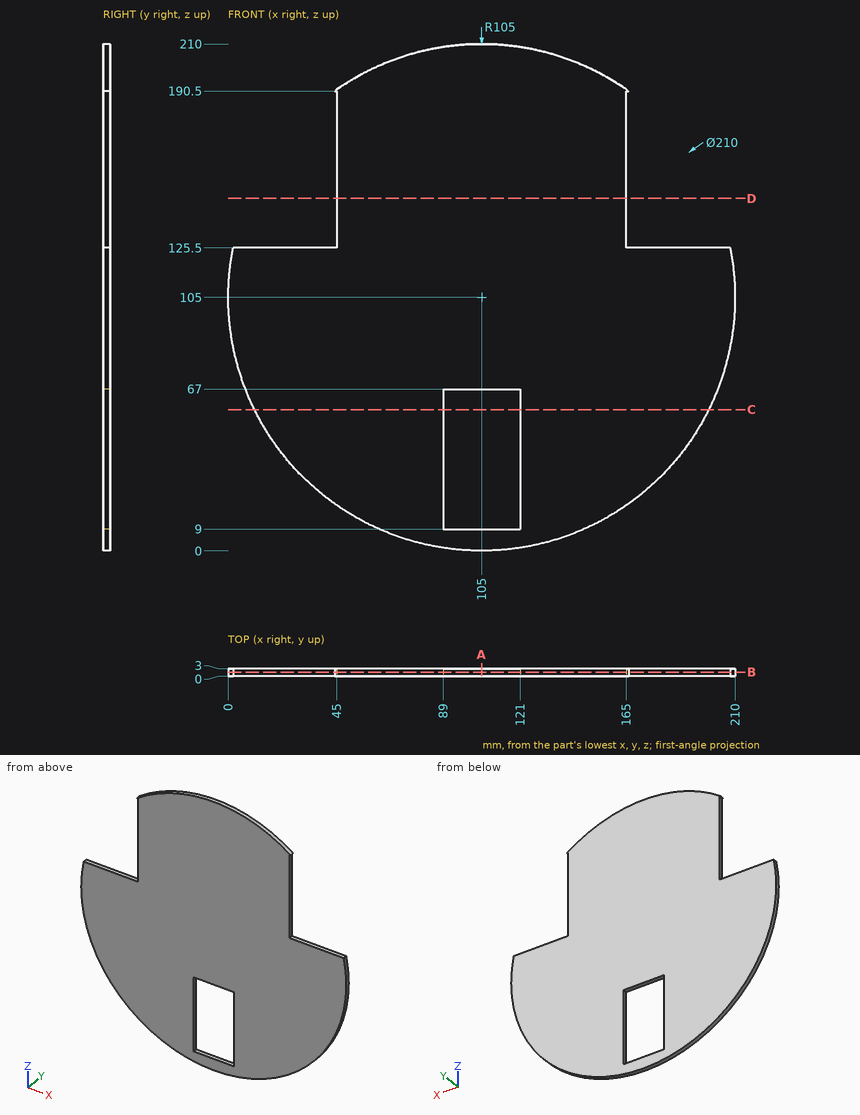
Input: dimensioned drawing with shaded views. Units: mm. Origin: part minimum x, y, z. Coordinates: 2 decimals unless noted, no trailing zeros. Order: outer loops, then holes, each group sorted by start corner. A loop starts at its lowest first (then second) coordinate and runs counter-clockwise, first axis right, second up. Notation, with made-up numbers: M 21.25,13.25 L 62.25,13.25 A25 ccw 62.25,34.25 Z; hole C 88.5,41.25 d6. An arc over 180 degrees is marked long. Write each question's results on one line, items separated by ' | '. Start each with the question number.
Item 1: Cut plane B-B (y = 1.6). Return loops of the section in (x, z).
Item 2: Cut plane C-C (z = 58.5). Return loops of the section in (x, y), and give its area (3 significant figures).
Item 3: First-contact query: pin 1 Ø1.5 at (y, z) = (0.5, 41.5) entering from -X; pin 2 Ø1.5 at (x, y) = (191.5, 1) entering from +Z; pin 3 Ø6 at (x, z) = (42, 86.5) entering from -Y; pin 4 Ø0.9 at (y, z) = (2, 47.5) entering from -X. Flat tips, straight axial feed; report the tip coordinate or a pass-through.
Item 4: Line query: probe 1 along Z at (x, y) = (106.5, 1.1); probe 2 along X at (y, z) = (2.2, 50.5); probe 3 along X at (y, z) = (1.5, 54). Output: solid intervals per line, ascending.
Item 5: Cut plane D-D (z = 146). Return loops of the section in (x, y).
Item 6: Cut plane A-A (x = 105). Return loops of the section in (y, z).
Checked values:
1) outline: M 2.02,125.5 A105 ccw long 207.98,125.5 L 165,125.5 L 165,190.5 L 165.95,190.5 A105 ccw 44.05,190.5 L 45,190.5 L 45,125.5 Z; hole M 89,9 L 121,9 L 121,67 L 89,67 Z
2) outline: M 10.86,0 L 89,0 L 89,3 L 10.86,3 Z; M 121,0 L 199.14,0 L 199.14,3 L 121,3 Z | area: 469 mm2
3) pin 1: stops at x = 20.81 | pin 2: stops at z = 125.5 | pin 3: stops at y = 0 | pin 4: stops at x = 16.85
4) probe 1: z = 0.01 to 9, 67 to 209.99 | probe 2: x = 15.25 to 89, 121 to 194.75 | probe 3: x = 13.22 to 89, 121 to 196.78
5) outline: M 45,0 L 165,0 L 165,3 L 45,3 Z
6) outline: M 0,0 L 3,0 L 3,9 L 0,9 Z; M 0,67 L 3,67 L 3,210 L 0,210 Z
